```python
from build123d import *

# Parameters (mm, degrees)
MODEL_W             = 6
MODEL_H             = 6
BOSS_EXTRUDE1_DEPTH = 6


with BuildPart() as part:
    # Model → Boss-Extrude1 (new body)
    with BuildSketch(Plane.XY):
        with BuildLine():
            Line((3463.892984012, 1061.748947436), (3473.892984012, 1061.748947436))
            Line((3473.892984012, 1061.748947436), (3473.892984012, 1055.748947436))
            Line((3473.892984012, 1055.748947436), (3479.892984012, 1055.748947436))
            Line((3479.892984012, 1055.748947436), (3479.892984012, 1061.748947436))
            Line((3479.892984012, 1061.748947436), (3491.892984012, 1061.748947436))
            Line((3491.892984012, 1061.748947436), (3506.94434904, 1061.748947436))
            ThreePointArc((3506.94434904, 1061.748947436), (3463.94434904, 1104.748947436), (3420.94434904, 1061.748947436))
            Line((3420.94434904, 1061.748947436), (3435.892984012, 1061.748947436))
            Line((3435.892984012, 1061.748947436), (3435.892984012, 1055.748947436))
            Line((3435.892984012, 1055.748947436), (3441.892984012, 1055.748947436))
            Line((3441.892984012, 1055.748947436), (3441.892984012, 1061.748947436))
            Line((3441.892984012, 1061.748947436), (3463.892984012, 1061.748947436))
        make_face()
        with Locations((3476.94434904, 1074.748947436)):
            Rectangle(MODEL_W, MODEL_H, mode=Mode.SUBTRACT)
        with Locations((3450.94434904, 1074.748947436)):
            Rectangle(MODEL_W, MODEL_H, mode=Mode.SUBTRACT)
        with Locations((3463.94434904, 1080.748947436)):
            Rectangle(MODEL_W, MODEL_H, mode=Mode.SUBTRACT)
        with Locations((3463.94434904, 1068.57340627)):
            Rectangle(MODEL_W, MODEL_H, mode=Mode.SUBTRACT)
    extrude(amount=BOSS_EXTRUDE1_DEPTH)


solid = part.part
```
Can you work these out from the model? Positions are in its coordinate system, mm. A direction names the side the tool comes from. Give positions to 0.01 mm unless a question says otherwise; leave off trailing zeros. Loops run counter-clockwise (first coordinate to the right, second up) from the corner with the lowest first, then second, coordinate; pieces in that order, holes last. Notation, with made-up numbers: M -18,-24 L 33,-24 A27 ccw 33,8 Z; hole C -11.5,-12.75 d6. An arc over 180 degrees is marked long. One line per item, written item: value.
(1) I need wall thicknesses on line 1 (Y direction, x = 3466, z = 2.5); line 2 (X direction, y = 1075.5, z = 0.9); line 3 (Y direction, x = 3453, z = 3.65). Which ranges of each line are inside material? Lowest first, please.
Returned:
line 1: 1061.75 to 1065.57, 1071.57 to 1077.75, 1083.75 to 1104.7
line 2: 3423.2 to 3447.94, 3453.94 to 3473.94, 3479.94 to 3504.69
line 3: 1061.75 to 1071.75, 1077.75 to 1103.33
(2) Suppose I cut it at B-B on x = 3475.5. List the corners of the cut face in (y, z) for me.
Returned:
outline: M 1055.75,0 L 1071.75,0 L 1071.75,6 L 1055.75,6 Z; M 1077.75,0 L 1103.17,0 L 1103.17,6 L 1077.75,6 Z
(3) We'd pull the mould along X, two halves only. Please class faces 5 (the face through (3441.893, 1059, 3)), 6 (the face through (3479.944, 1075, 3)), 7 (the face through (3435.893, 1059, 3)), 8 (the face through (3463, 1075, 6)): released by +X, released by -X, zero draft, split by the parting line, or undercut.
Returned:
face 5: undercut
face 6: undercut
face 7: released by -X
face 8: zero draft
(4) Suppose I cut it at A-A on z = 0.95. List the corners of the cut face in (x, y) for me.
Returned:
outline: M 3420.94,1061.75 L 3435.89,1061.75 L 3435.89,1055.75 L 3441.89,1055.75 L 3441.89,1061.75 L 3473.89,1061.75 L 3473.89,1055.75 L 3479.89,1055.75 L 3479.89,1061.75 L 3506.94,1061.75 A43 ccw Z; hole M 3447.94,1071.75 L 3453.94,1071.75 L 3453.94,1077.75 L 3447.94,1077.75 Z; hole M 3460.94,1065.57 L 3466.94,1065.57 L 3466.94,1071.57 L 3460.94,1071.57 Z; hole M 3460.94,1077.75 L 3466.94,1077.75 L 3466.94,1083.75 L 3460.94,1083.75 Z; hole M 3473.94,1071.75 L 3479.94,1071.75 L 3479.94,1077.75 L 3473.94,1077.75 Z
(5) Which directions (+Z, -Z, +X, -X, +Y, -Y) give clear straight access to the entire face, cutting with the end or side of a thin tool? Please do faces 1 (the face through (3466.944, 1069, 3)), 2 (the face through (3493, 1061.749, 3)), 3 (the face through (3473.893, 1059, 3)), 4 (the face through (3428, 1061.749, 3)).
Returned:
face 1: +Z, -Z
face 2: +Z, -Z, +X, -Y
face 3: +Z, -Z, -Y
face 4: +Z, -Z, -X, -Y
(6) Suppose I cut it at D-D on x = 3432. List the corners of the cut face in (y, z) for me, plus the area to 3 significant figures.
Returned:
outline: M 1061.75,0 L 1090.53,0 L 1090.53,6 L 1061.75,6 Z
area: 173 mm^2
(7) Suppose I cut it at C-C on y = 1081. List the corners of the cut face in (x, z) for me.
Returned:
outline: M 3425.49,0 L 3460.94,0 L 3460.94,6 L 3425.49,6 Z; M 3466.94,0 L 3502.39,0 L 3502.39,6 L 3466.94,6 Z
(8) Will these pins go through, and if not, where does the flat tip stop? pin 1 (2 mm diameter, centred on x = 3494.5, z = 3.5, fed in from +Y); pin 2 (3 mm diameter, centred on y = 1058, z = 2.5, fed in from -X); pin 3 (1.8 mm diameter, centred on x = 3464.5, z = 4, fed in from -Y).
Returned:
pin 1: y = 1092.98
pin 2: x = 3435.89
pin 3: y = 1061.75
